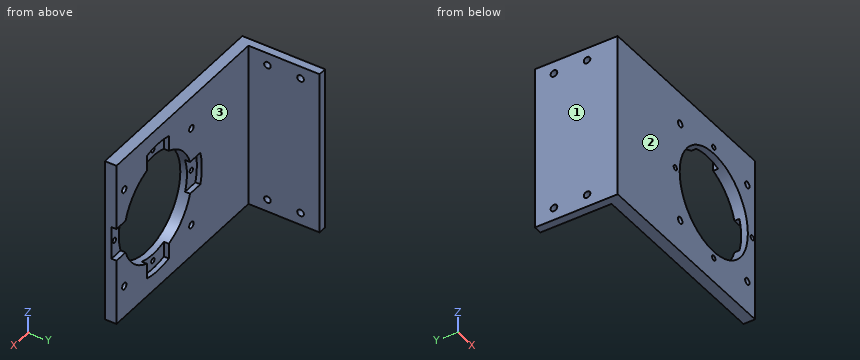
from build123d import *

# Parameters (mm, degrees)
BOSS_EXTRUDE1_DEPTH = 100
CUT_EXTRUDE1_REACH  = 167.753
SKETCH2_R           = 31
SKETCH2_R_2         = 2
CUT_EXTRUDE2_REACH  = 166.012
SKETCH3_R           = 2
CUT_EXTRUDE3_DEPTH  = 3
CUT_EXTRUDE4_REACH  = 168.556
SKETCH6_R           = 1.5


with BuildPart() as part:
    # Sketch1 → Boss-Extrude1 (new body)
    with BuildSketch(Plane.XY):
        Polygon((0, 0), (125, 0), (125, 7), (5, 7), (5, 50), (0, 50), align=None)
    extrude(amount=BOSS_EXTRUDE1_DEPTH)

    # Sketch2 → Cut-Extrude1 (cut, up to next)
    with BuildSketch(Plane(origin=(0, 7, 0), x_dir=(1, 0, 0), z_dir=(0, 1, 0)), mode=Mode.PRIVATE) as cut_extrude1_sk1:
        with Locations(Location((87.42, -50, 0), (0, 0, 180))):
            Circle(SKETCH2_R)
    cut_extrude1_tool1 = extrude(cut_extrude1_sk1.sketch, amount=-CUT_EXTRUDE1_REACH, mode=Mode.PRIVATE) & part.part
    # Sketch2 → Cut-Extrude1 (cut, up to next)
    with BuildSketch(Plane(origin=(0, 7, 0), x_dir=(1, 0, 0), z_dir=(0, 1, 0)), mode=Mode.PRIVATE) as cut_extrude1_sk2:
        with Locations(Location((56.92, -19.5, 0), (0, 0, 180))):
            Circle(SKETCH2_R_2)
    cut_extrude1_tool2 = extrude(cut_extrude1_sk2.sketch, amount=-CUT_EXTRUDE1_REACH, mode=Mode.PRIVATE) & part.part
    # Sketch2 → Cut-Extrude1 (cut, up to next)
    with BuildSketch(Plane(origin=(0, 7, 0), x_dir=(1, 0, 0), z_dir=(0, 1, 0)), mode=Mode.PRIVATE) as cut_extrude1_sk3:
        with Locations(Location((56.92, -80.5, 0), (0, 0, 270))):
            Circle(SKETCH2_R_2)
    cut_extrude1_tool3 = extrude(cut_extrude1_sk3.sketch, amount=-CUT_EXTRUDE1_REACH, mode=Mode.PRIVATE) & part.part
    # Sketch2 → Cut-Extrude1 (cut, up to next)
    with BuildSketch(Plane(origin=(0, 7, 0), x_dir=(1, 0, 0), z_dir=(0, 1, 0)), mode=Mode.PRIVATE) as cut_extrude1_sk4:
        with Locations(Location((117.92, -19.5, 0), (0, 0, 270))):
            Circle(SKETCH2_R_2)
    cut_extrude1_tool4 = extrude(cut_extrude1_sk4.sketch, amount=-CUT_EXTRUDE1_REACH, mode=Mode.PRIVATE) & part.part
    # Sketch2 → Cut-Extrude1 (cut, up to next)
    with BuildSketch(Plane(origin=(0, 7, 0), x_dir=(1, 0, 0), z_dir=(0, 1, 0)), mode=Mode.PRIVATE) as cut_extrude1_sk5:
        with Locations(Location((117.92, -80.5, 0), (0, 0, 180))):
            Circle(SKETCH2_R_2)
    cut_extrude1_tool5 = extrude(cut_extrude1_sk5.sketch, amount=-CUT_EXTRUDE1_REACH, mode=Mode.PRIVATE) & part.part
    add(cut_extrude1_tool1.solids().sort_by_distance((87.42, 7, 50))[0], mode=Mode.SUBTRACT)
    add(cut_extrude1_tool2.solids().sort_by_distance((56.92, 7, 19.5))[0], mode=Mode.SUBTRACT)
    add(cut_extrude1_tool3.solids().sort_by_distance((56.92, 7, 80.5))[0], mode=Mode.SUBTRACT)
    add(cut_extrude1_tool4.solids().sort_by_distance((117.92, 7, 19.5))[0], mode=Mode.SUBTRACT)
    add(cut_extrude1_tool5.solids().sort_by_distance((117.92, 7, 80.5))[0], mode=Mode.SUBTRACT)

    # Sketch3 → Cut-Extrude2 (cut, up to next)
    with BuildSketch(Plane(origin=(5, 0, 0), x_dir=(0, 0, -1), z_dir=(1, 0, 0)), mode=Mode.PRIVATE) as cut_extrude2_sk1:
        with Locations((-92.5, 38.5)):
            Circle(SKETCH3_R)
    cut_extrude2_tool1 = extrude(cut_extrude2_sk1.sketch, amount=-CUT_EXTRUDE2_REACH, mode=Mode.PRIVATE) & part.part
    # Sketch3 → Cut-Extrude2 (cut, up to next)
    with BuildSketch(Plane(origin=(5, 0, 0), x_dir=(0, 0, -1), z_dir=(1, 0, 0)), mode=Mode.PRIVATE) as cut_extrude2_sk2:
        with Locations(Location((-92.5, 18.5, 0), (0, 0, 90))):
            Circle(SKETCH3_R)
    cut_extrude2_tool2 = extrude(cut_extrude2_sk2.sketch, amount=-CUT_EXTRUDE2_REACH, mode=Mode.PRIVATE) & part.part
    # Sketch3 → Cut-Extrude2 (cut, up to next)
    with BuildSketch(Plane(origin=(5, 0, 0), x_dir=(0, 0, -1), z_dir=(1, 0, 0)), mode=Mode.PRIVATE) as cut_extrude2_sk3:
        with Locations(Location((-7.5, 38.5, 0), (0, 0, 90))):
            Circle(SKETCH3_R)
    cut_extrude2_tool3 = extrude(cut_extrude2_sk3.sketch, amount=-CUT_EXTRUDE2_REACH, mode=Mode.PRIVATE) & part.part
    # Sketch3 → Cut-Extrude2 (cut, up to next)
    with BuildSketch(Plane(origin=(5, 0, 0), x_dir=(0, 0, -1), z_dir=(1, 0, 0)), mode=Mode.PRIVATE) as cut_extrude2_sk4:
        with Locations((-7.5, 18.5)):
            Circle(SKETCH3_R)
    cut_extrude2_tool4 = extrude(cut_extrude2_sk4.sketch, amount=-CUT_EXTRUDE2_REACH, mode=Mode.PRIVATE) & part.part
    add(cut_extrude2_tool1.solids().sort_by_distance((5, 38.5, 92.5))[0], mode=Mode.SUBTRACT)
    add(cut_extrude2_tool2.solids().sort_by_distance((5, 18.5, 92.5))[0], mode=Mode.SUBTRACT)
    add(cut_extrude2_tool3.solids().sort_by_distance((5, 38.5, 7.5))[0], mode=Mode.SUBTRACT)
    add(cut_extrude2_tool4.solids().sort_by_distance((5, 18.5, 7.5))[0], mode=Mode.SUBTRACT)

    # Sketch4 → Cut-Extrude3 (cut)
    with BuildSketch(Plane(origin=(0, 7, 0), x_dir=(1, 0, 0), z_dir=(0, 1, 0))):
        with BuildLine():
            Line((97.42, -20.657198498), (97.42, -11.270166538))
            ThreePointArc((97.42, -11.270166538), (87.42, -10), (77.42, -11.270166538))
            Line((77.42, -11.270166538), (77.42, -20.657198498))
            ThreePointArc((77.42, -20.657198498), (87.42, -19), (97.42, -20.657198498))
        make_face()
        with BuildLine():
            Line((116.762801502, -60), (126.149833462, -60))
            ThreePointArc((126.149833462, -60), (127.42, -50), (126.149833462, -40))
            Line((126.149833462, -40), (116.762801502, -40))
            ThreePointArc((116.762801502, -40), (118.42, -50), (116.762801502, -60))
        make_face()
        with BuildLine():
            Line((77.42, -79.342801502), (77.42, -88.729833462))
            ThreePointArc((77.42, -88.729833462), (87.42, -90), (97.42, -88.729833462))
            Line((97.42, -88.729833462), (97.42, -79.342801502))
            ThreePointArc((97.42, -79.342801502), (87.42, -81), (77.42, -79.342801502))
        make_face()
        with BuildLine():
            Line((58.077198498, -40), (48.690166538, -40))
            ThreePointArc((48.690166538, -40), (47.42, -50), (48.690166538, -60))
            Line((48.690166538, -60), (58.077198498, -60))
            ThreePointArc((58.077198498, -60), (56.42, -50), (58.077198498, -40))
        make_face()
    extrude(amount=-CUT_EXTRUDE3_DEPTH, mode=Mode.SUBTRACT)

    # Sketch6 → Cut-Extrude4 (cut, up to next)
    with BuildSketch(Plane(origin=(0, 4, 0), x_dir=(1, 0, 0), z_dir=(0, 1, 0)), mode=Mode.PRIVATE) as cut_extrude4_sk1:
        with Locations(Location((87.42, -15, 0), (0, 0, 180))):
            Circle(SKETCH6_R)
    cut_extrude4_tool1 = extrude(cut_extrude4_sk1.sketch, amount=-CUT_EXTRUDE4_REACH, mode=Mode.PRIVATE) & part.part
    # Sketch6 → Cut-Extrude4 (cut, up to next)
    with BuildSketch(Plane(origin=(0, 4, 0), x_dir=(1, 0, 0), z_dir=(0, 1, 0)), mode=Mode.PRIVATE) as cut_extrude4_sk2:
        with Locations(Location((122.42, -50, 0), (0, 0, 180))):
            Circle(SKETCH6_R)
    cut_extrude4_tool2 = extrude(cut_extrude4_sk2.sketch, amount=-CUT_EXTRUDE4_REACH, mode=Mode.PRIVATE) & part.part
    # Sketch6 → Cut-Extrude4 (cut, up to next)
    with BuildSketch(Plane(origin=(0, 4, 0), x_dir=(1, 0, 0), z_dir=(0, 1, 0)), mode=Mode.PRIVATE) as cut_extrude4_sk3:
        with Locations(Location((87.42, -85, 0), (0, 0, 180))):
            Circle(SKETCH6_R)
    cut_extrude4_tool3 = extrude(cut_extrude4_sk3.sketch, amount=-CUT_EXTRUDE4_REACH, mode=Mode.PRIVATE) & part.part
    # Sketch6 → Cut-Extrude4 (cut, up to next)
    with BuildSketch(Plane(origin=(0, 4, 0), x_dir=(1, 0, 0), z_dir=(0, 1, 0)), mode=Mode.PRIVATE) as cut_extrude4_sk4:
        with Locations(Location((52.42, -50, 0), (0, 0, 180))):
            Circle(SKETCH6_R)
    cut_extrude4_tool4 = extrude(cut_extrude4_sk4.sketch, amount=-CUT_EXTRUDE4_REACH, mode=Mode.PRIVATE) & part.part
    add(cut_extrude4_tool1.solids().sort_by_distance((87.42, 4, 15))[0], mode=Mode.SUBTRACT)
    add(cut_extrude4_tool2.solids().sort_by_distance((122.42, 4, 50))[0], mode=Mode.SUBTRACT)
    add(cut_extrude4_tool3.solids().sort_by_distance((87.42, 4, 85))[0], mode=Mode.SUBTRACT)
    add(cut_extrude4_tool4.solids().sort_by_distance((52.42, 4, 50))[0], mode=Mode.SUBTRACT)


solid = part.part
Work out the finished part from the listing and answer in its coordinate system (mm). Face numbers are marked on the shaded views. Coordinates: 2 decimals unless noted, no trailing zeros. Write each loop counter-clockwise with the first axis right and the second up, starting at its lowest first coordinate (ties: lowest second). Pieces come first, ordered by that corner, then holes.
1. For a pull along Y with two mould halves and no side action, classify the marked faces 1, 2 and 3 as +Y half, -Y half, draft (parallel to the pull), parting line (faces both ways), or undercut.
Results list:
face 1: draft
face 2: -Y half
face 3: +Y half
2. The part is cut by section C-C, the plane z = 92.5. Write down the section's boundary in (x, y), and give its area (3 significant figures).
Results list:
outline: (0, 0) - (125, 0) - (125, 7) - (5, 7) - (5, 16.5) - (0, 16.5) - close; (0, 20.5) - (5, 20.5) - (5, 36.5) - (0, 36.5) - close; (0, 40.5) - (5, 40.5) - (5, 50) - (0, 50) - close
area: 1,050 mm2
3. The part is cut by section A-A, the plane z = 50. Write down the section's boundary in (x, y), and give its area (3 significant figures).
Results list:
outline: (0, 0) - (50.92, 0) - (50.92, 4) - (47.42, 4) - (47.42, 7) - (5, 7) - (5, 50) - (0, 50) - close; (53.92, 0) - (56.42, 0) - (56.42, 4) - (53.92, 4) - close; (118.42, 0) - (120.92, 0) - (120.92, 4) - (118.42, 4) - close; (123.92, 0) - (125, 0) - (125, 4) - (123.92, 4) - close
area: 585 mm2
4. The part is cut by section D-D, the plane z = 15. Write down the section's boundary in (x, y), and give its area (3 significant figures).
Results list:
outline: (0, 0) - (85.92, 0) - (85.92, 4) - (77.42, 4) - (77.42, 7) - (5, 7) - (5, 50) - (0, 50) - close; (88.92, 0) - (125, 0) - (125, 7) - (97.42, 7) - (97.42, 4) - (88.92, 4) - close
area: 1,020 mm2
5. Flat-ended cylindrical pins translate along their axes: pin 1 (6.5 mm diameter, centred on x = 56.92, z = 19.5, fed in from +Y); pin 2 (9 mm diameter, centred on x = 120.5, z = 45.5, fed in from +Y); pin 3 (8 mm diameter, centred on y = 39, z = 83.5, fed in from +X). Find the tip coordinate at first contact, or state that the pin passes through.
Results list:
pin 1: stops at y = 7
pin 2: stops at y = 4
pin 3: stops at x = 5
6. The part is cut by section B-B, the plane x = 110. Write down the section's boundary in (y, z), and give its area (3 significant figures).
Results list:
outline: (0, 0) - (7, 0) - (7, 28.76) - (0, 28.76) - close; (0, 71.24) - (7, 71.24) - (7, 100) - (0, 100) - close
area: 403 mm2
7. Consider line 1 along Z through (x, y) = (87.42, 2.8); line 2 along Z through (x, y) = (87, 2); line 3 along Y through (x, z) = (2, 92). Determine where each line is inside the solid, lowest interval first.
Results list:
line 1: z = 0 to 13.5, 16.5 to 19, 81 to 83.5, 86.5 to 100
line 2: z = 0 to 13.56, 16.44 to 19, 81 to 83.56, 86.44 to 100
line 3: y = 0 to 16.56, 20.44 to 36.56, 40.44 to 50
